CAD build for the part. Positions are in the model's coordinates, mm. Coordinates: 2 decimals unless noted, no trailing zeros. Write each loop counter-clockwise with the first axis right and the second up, starting at its lowest first coordinate (ties: lowest second). Pieces come first, ordered by that corner, then holes. Notation, with made-up numbers: (88.25, 55) -> (120.25, 55) arc R24 ccw to (120.25, 69) -> close; hole circle Ø8 at (21.5, 63). An arc over 180 degrees is marked (long way). Answer as CSV lines item,"result".
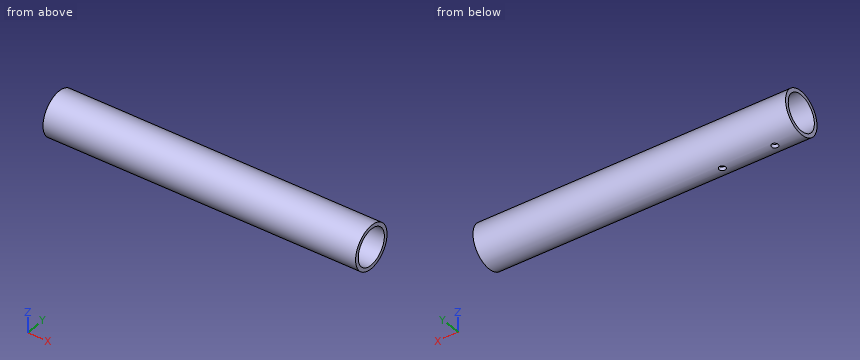
```python
from build123d import *

# Parameters (mm, degrees)
SKETCH1_R                = 21.082
SKETCH1_R_2              = 17.526
BOSS_EXTRUDE1_DEPTH      = 127
BOSS_EXTRUDE1_DEPTH_BACK = 174.625
SKETCH2_R                = 3.175
CUT_EXTRUDE1_DEPTH       = 22.082


with BuildPart() as part:
    # Sketch1 → Boss-Extrude1 (new body, two sides)
    with BuildSketch(Plane(origin=(0, 0, 0), x_dir=(0, 0, -1), z_dir=(1, 0, 0))) as boss_extrude1_sk:
        Circle(SKETCH1_R)
        Circle(SKETCH1_R_2, mode=Mode.SUBTRACT)
    extrude(amount=BOSS_EXTRUDE1_DEPTH)
    extrude(boss_extrude1_sk.sketch, amount=-BOSS_EXTRUDE1_DEPTH_BACK)

    # Sketch2 → Cut-Extrude1 (cut, through all)
    with BuildSketch(Plane.XY):
        with Locations((-98.425, 0)):
            Circle(SKETCH2_R)
        with Locations((-149.225, 0)):
            Circle(SKETCH2_R)
    extrude(amount=-CUT_EXTRUDE1_DEPTH, mode=Mode.SUBTRACT)


solid = part.part
```
Item 1: Saw through at A-A on y = 0. Give the cut face in (x, z) (3 decimals).
Answer below:
outline,"(-174.625, -21.082) -> (-152.4, -21.082) -> (-152.4, -17.526) -> (-174.625, -17.526) -> close; (-174.625, 17.526) -> (127, 17.526) -> (127, 21.082) -> (-174.625, 21.082) -> close; (-146.05, -21.082) -> (-101.6, -21.082) -> (-101.6, -17.526) -> (-146.05, -17.526) -> close; (-95.25, -21.082) -> (127, -21.082) -> (127, -17.526) -> (-95.25, -17.526) -> close"
Item 2: Flat gauge pins, fed straight in: pin 1 (10 mm diameter, centred on x = -55, z = 12, fed in from -Y); pin 2 (1.5 mm diameter, centred on x = -18, z = 16.5, fed in from -Y); pin 3 (8 mm diameter, centred on x = -65.5, y = -5, fed in from +Z). Where does each tip first touch, or does it go through?
Answer below:
pin 1,"stops at y = -19.89"
pin 2,"stops at y = -14.01"
pin 3,"stops at z = 21.06"
Item 3: Saw through at C-C on y = -11. Give the cut face in (x, z) (3 decimals).
Answer below:
outline,"(-174.625, -17.985) -> (127, -17.985) -> (127, -13.644) -> (-174.625, -13.644) -> close; (-174.625, 13.644) -> (127, 13.644) -> (127, 17.985) -> (-174.625, 17.985) -> close"
Item 4: Saw through at D-D on x = 90.5. Give the cut face in (y, z), and give its area (3 significant figures).
Answer below:
outline,"circle Ø42.16 at (0, 0); hole circle Ø35.05 at (0, 0)"
area,"431 mm2"
Item 5: Wall check: line 1 (X direction, y = 0, z = -18) (3 decimals); line 2 (Y direction, x = 101, z = 0); line 3 (Y direction, x = 84, z = 9.5). Give the ranges that are in metal, low to high. Write a range as from..to.
Answer below:
line 1,"x = -174.625..-152.4, -146.05..-101.6, -95.25..127"
line 2,"y = -21.08..-17.53, 17.53..21.08"
line 3,"y = -18.82..-14.73, 14.73..18.82"
Item 6: Saw through at B-B on z = 0. Give the cut face in (x, y) (3 decimals).
Answer below:
outline,"(-174.625, -21.082) -> (127, -21.082) -> (127, -17.526) -> (-174.625, -17.526) -> close; (-174.625, 17.526) -> (127, 17.526) -> (127, 21.082) -> (-174.625, 21.082) -> close"
